```python
from build123d import *

# Parameters (mm, degrees)
BOSS_EXTRUDE2_DEPTH   = 58.42
BOSS_EXTRUDE2_2_DEPTH = 58.42
BOSS_EXTRUDE3_DEPTH   = 7.62
SKETCH6_W             = 73.66
SKETCH6_H             = 76.2
SKETCH6_W_2           = 70.104
SKETCH6_H_2           = 72.644
SKETCH6_W_3           = 63.5
SKETCH6_H_3           = 66.04
SKETCH6_W_4           = 58.42
SKETCH6_H_4           = 60.96
BOSS_EXTRUDE4_DEPTH   = 25.4
SKETCH7_W             = 73.66
SKETCH7_H             = 76.2
SKETCH7_W_2           = 70.104
SKETCH7_H_2           = 72.644
SKETCH7_W_3           = 63.5
SKETCH7_H_3           = 66.04
SKETCH7_W_4           = 58.42
SKETCH7_H_4           = 60.96
BOSS_EXTRUDE5_DEPTH   = 25.4
CHAMFER1_SIZE         = 2.773453185
CHAMFER1_SIZE_2       = 7.62
CUT_EXTRUDE3_REACH    = 158.41
SKETCH10_W            = 25.4
SKETCH10_H            = 177.72143494
SKETCH11_R            = 4.064
SKETCH11_R_2          = 2.5
BOSS_EXTRUDE6_DEPTH   = 10
SKETCH12_R            = 17
CUT_EXTRUDE4_DEPTH    = 6.5


with BuildPart() as part:
    # Sketch3 → Boss-Extrude2 (new body)
    with BuildSketch(Plane(origin=(0, 0, 0), x_dir=(0, 0, -1), z_dir=(1, 0, 0))):
        with BuildLine():
            Line((-62.063264719, -88.6355278), (-66.433917164, -94.877466378))
            ThreePointArc((-66.433917164, -94.877466378), (10.094726748, -115.383254712), (81.899935824, -81.899935824))
            Line((81.899935824, -81.899935824), (76.511782152, -76.511782152))
            ThreePointArc((76.511782152, -76.511782152), (9.430599988, -107.792251112), (-62.063264719, -88.6355278))
        make_face()
    extrude(amount=BOSS_EXTRUDE2_DEPTH)



with BuildPart() as body_2:
    # Sketch3 → Boss-Extrude2 2 (new body)
    with BuildSketch(Plane(origin=(0, 0, 0), x_dir=(0, 0, -1), z_dir=(1, 0, 0))):
        with BuildLine():
            ThreePointArc((28.018399098, -28.018399098), (3.453459151, -39.473218717), (-22.727392714, -32.458080603))
            Line((-22.727392714, -32.458080603), (-27.098045159, -38.70001918))
            ThreePointArc((-27.098045159, -38.70001918), (4.11758591, -47.064222317), (33.40655277, -33.40655277))
            Line((33.40655277, -33.40655277), (28.018399098, -28.018399098))
        make_face()
    extrude(amount=BOSS_EXTRUDE2_2_DEPTH)


with BuildPart() as part_1:
    add(part.part)

    add(body_2.part)  # Boss-Extrude3 merges body 2
    # Sketch4 → Boss-Extrude3 (add)
    with BuildSketch(Plane(origin=(58.42, 0, 0), x_dir=(0, 0, -1), z_dir=(1, 0, 0))):
        with BuildLine():
            Line((-22.727392714, -32.458080603), (-66.433917164, -94.877466378))
            ThreePointArc((-66.433917164, -94.877466378), (10.094726748, -115.383254712), (81.899935824, -81.899935824))
            Line((81.899935824, -81.899935824), (28.018399098, -28.018399098))
            ThreePointArc((28.018399098, -28.018399098), (3.453459151, -39.473218717), (-22.727392714, -32.458080603))
        make_face()
    boss_extrude3 = extrude(amount=BOSS_EXTRUDE3_DEPTH)

    # Mirror1: Boss-Extrude3 across plane
    add(boss_extrude3.mirror(Plane.ZY.offset(-29.21)))

    # Sketch6 → Boss-Extrude4 (add)
    # profile 1 of 2: a face of its own
    with BuildSketch(Plane(origin=(0, 0, 0), x_dir=(1, 0, 0), z_dir=(0, 0.5735764363510462, 0.8191520442889917))):
        with Locations((29.21, -77.724)):
            Rectangle(SKETCH6_W, SKETCH6_H)
        with Locations((29.21, -77.724)):
            Rectangle(SKETCH6_W_2, SKETCH6_H_2, mode=Mode.SUBTRACT)
    # profile 2 of 2: a face of its own
    with BuildSketch(Plane(origin=(0, 0, 0), x_dir=(1, 0, 0), z_dir=(0, 0.5735764363510462, 0.8191520442889917))):
        with Locations((29.21, -77.724)):
            Rectangle(SKETCH6_W_3, SKETCH6_H_3)
        with Locations((29.21, -77.724)):
            Rectangle(SKETCH6_W_4, SKETCH6_H_4, mode=Mode.SUBTRACT)
    extrude(amount=BOSS_EXTRUDE4_DEPTH)

    # Sketch7 → Boss-Extrude5 (add)
    # profile 1 of 2: a face of its own
    with BuildSketch(Plane(origin=(0, 0, 0), x_dir=(1, 0, 0), z_dir=(0, 0.7071067811865503, -0.7071067811865447))):
        with Locations((29.21, 77.724)):
            Rectangle(SKETCH7_W, SKETCH7_H)
        with Locations((29.21, 77.724)):
            Rectangle(SKETCH7_W_2, SKETCH7_H_2, mode=Mode.SUBTRACT)
    # profile 2 of 2: a face of its own
    with BuildSketch(Plane(origin=(0, 0, 0), x_dir=(1, 0, 0), z_dir=(0, 0.7071067811865503, -0.7071067811865447))):
        with Locations((29.21, 77.724)):
            Rectangle(SKETCH7_W_3, SKETCH7_H_3)
        with Locations((29.21, 77.724)):
            Rectangle(SKETCH7_W_4, SKETCH7_H_4, mode=Mode.SUBTRACT)
    extrude(amount=BOSS_EXTRUDE5_DEPTH)

    # Chamfer1
    # the kernel refuses this chamfer: 7.62, 2.773453185 mm, written as the material it takes off along each edge
    with BuildSketch(Plane(origin=(58.42, -15.446040528, -51.367065013), x_dir=(0, 0.7736626875489875, 0.6335977003544738), z_dir=(-1, 0, 0)), Plane(origin=(0, -24.131177697, 47.904507084), x_dir=(0, 0.8719320989550161, -0.489626811778011), z_dir=(1, 0, 0))) as chamfer1_piece_1:
        Polygon((CHAMFER1_SIZE * 0.995083363221, -CHAMFER1_SIZE * 0.0990409022559), (-CHAMFER1_SIZE_2 * 0.0990409022521, -CHAMFER1_SIZE_2 * 0.995083363182), (0, 0), align=None)
    extrude(amount=58.42, mode=Mode.SUBTRACT)
    with BuildSketch(Plane(origin=(0, -58.551269909, -94.472294394), x_dir=(0, -0.6977227871251116, 0.7163678610367485), z_dir=(1, 0, 0)), Plane(origin=(58.42, -74.066686317, 82.869726644), x_dir=(0, -0.562726836605906, -0.8266429140587307), z_dir=(-1, 0, 0))) as chamfer1_piece_2:
        Polygon((CHAMFER1_SIZE_2 * 0.999913086528, CHAMFER1_SIZE_2 * 0.0131840581986), (-CHAMFER1_SIZE * 0.0131840581992, CHAMFER1_SIZE * 0.999913086567), (0, 0), align=None)
    extrude(amount=58.42, mode=Mode.SUBTRACT)

    # Sketch10 → Cut-Extrude3 (cut, up to next)
    with BuildSketch(Plane(origin=(0, -13.973562988, -1.22252835), x_dir=(-1, 0, 0), z_dir=(0, -0.9961946980917453, -0.08715574274766034)), mode=Mode.PRIVATE) as cut_extrude3_sk1:
        with Locations((-29.21, 6.675062398)):
            Rectangle(SKETCH10_W, SKETCH10_H)
    cut_extrude3_tool1 = extrude(cut_extrude3_sk1.sketch, amount=CUT_EXTRUDE3_REACH, mode=Mode.PRIVATE) & part_1.part
    add(cut_extrude3_tool1.solids().sort_by_distance((29.21, -13.391793, -7.87219))[0], mode=Mode.SUBTRACT)

    # Sketch11 → Boss-Extrude6 (add)
    with BuildSketch(Plane.ZY.offset(7.62)):
        with BuildLine():
            Line((-25.298191602, 2.271893855), (-28.018399098, -28.018399098))
            ThreePointArc((-28.018399098, -28.018399098), (-17.287205304, -35.654086845), (-4.646100514, -39.350668686))
            Line((-4.646100514, -39.350668686), (-3.089724987, -22.01997949))
            ThreePointArc((-3.089724987, -22.01997949), (1.526343902, -17.41376085), (6.873353249, -21.146699798))
            Line((6.873353249, -21.146699798), (11.420958182, -37.942365374))
            ThreePointArc((11.420958182, -37.942365374), (17.292970019, -35.651291196), (22.727392714, -32.458080603))
            Line((22.727392714, -32.458080603), (33.130623676, -25.173659861))
            Line((33.130623676, -25.173659861), (24.517199578, 6.638292315))
            ThreePointArc((24.517199578, 6.638292315), (-2.217847157, 25.302987057), (-25.298191602, 2.271893855))
        make_face()
        Circle(SKETCH11_R, mode=Mode.SUBTRACT)
        with Locations((-17.454015953, -10.75208478)):
            Circle(SKETCH11_R_2, mode=Mode.SUBTRACT)
        with Locations((17.454015953, 10.75208478)):
            Circle(SKETCH11_R_2, mode=Mode.SUBTRACT)
    extrude(amount=-BOSS_EXTRUDE6_DEPTH)

    # Sketch12 → Cut-Extrude4 (cut)
    with BuildSketch(Plane.ZY.offset(7.62)):
        Circle(SKETCH12_R)
    extrude(amount=-CUT_EXTRUDE4_DEPTH, mode=Mode.SUBTRACT)


solid = part_1.part
```
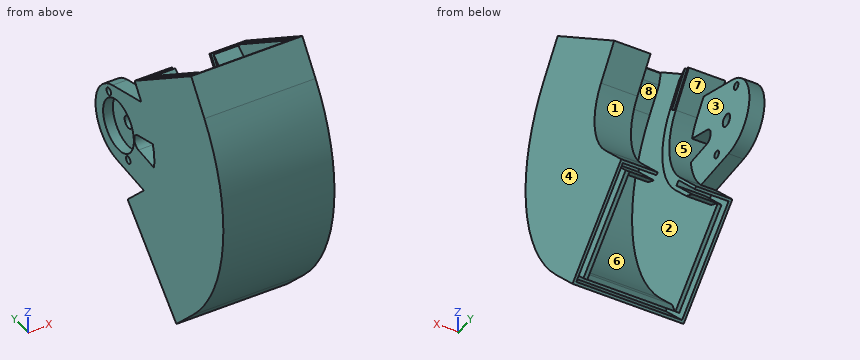
The model under review builds one solid part; all positions refer to its coordinate system, in mm. Face numbers are marked on the shaded views. A direction names the side the tool comes from. Give positions to 0.01 mm unless a question says otherwise; leave off trailing zeros. Write each loop counter-clockwise with the first axis right and the second up, starting at its lowest first coordinate (ties: lowest second). Pieces come first, ordered by that corner, then holes. Notation, with made-up numbers: M 65,-38 L 109,-38 A32 cw 109,-1 Z; hole C -10,72 d6. An arc over 180 degrees is marked long. Answer in a Markdown table with one row per item.
Item 1: Draft analysis for pull direction X (two halves, no side actions). For the marked faces 1, 2 and 3, state which applies: +X half, -X half, draft (parallel to the pull), parting line (faces both ways), or undercut.
Check sheet entries:
| item | result |
|---|---|
| face 1 | draft |
| face 2 | undercut |
| face 3 | +X half |
Item 2: Add section C-C on z = 0. Give the boundary of the cut face in (x, y).
Check sheet entries:
| item | result |
|---|---|
| outline | M -7.62,-115.82 L 66.04,-115.82 L 66.04,-39.62 L 41.91,-39.62 L 41.91,-47.24 L 58.42,-47.24 L 58.42,-108.2 L 0,-108.2 L 0,-47.24 L 16.51,-47.24 L 16.51,-39.62 L -7.62,-39.62 Z; M -7.62,-17.79 L 2.38,-17.79 L 2.38,-4.06 L -1.12,-4.06 L -1.12,-17 L -7.62,-17 Z; M -7.62,17 L -1.12,17 L -1.12,4.06 L 2.38,4.06 L 2.38,25.4 L -7.62,25.4 Z |
Item 3: Add section D-D on y = -103.5. Give the boundary of the cut face in (x, z).
Check sheet entries:
| item | result |
|---|---|
| outline | M -7.62,-51.99 L 66.04,-51.99 L 66.04,51.99 L -7.62,51.99 Z; hole M 0,-31.56 L 58.42,-31.56 L 58.42,31.56 L 0,31.56 Z |
Item 4: Add section B-B on y = 0. Give the boundary of the cut face in (x, z).
Check sheet entries:
| item | result |
|---|---|
| outline | M -7.62,-25.5 L 2.38,-25.5 L 2.38,-4.06 L -1.12,-4.06 L -1.12,-17 L -7.62,-17 Z; M -7.62,17 L -1.12,17 L -1.12,4.06 L 2.38,4.06 L 2.38,26.31 L -7.62,26.31 Z |
Item 5: For line 1 along X through (y, z) = (-35, -35.5); line 2 along X through (y, z) = (-94.5, 39); line 3 along Y through (x, z) = (-6, 0), list the stretches that pass through material, from the lowest coordinate up.
Check sheet entries:
| item | result |
|---|---|
| line 1 | -7.62 to -5.84, -2.54 to 0, 58.42 to 60.96, 64.26 to 66.04 |
| line 2 | -7.62 to 0, 58.42 to 66.04 |
| line 3 | -115.82 to -39.62, -17.79 to -17, 17 to 25.4 |
Item 6: Tool access review of the marked faces 4, 5, 6, 7 and 8: name each direction out of +Z, -Z, +X, -X, +Y, -Y from which nothing blocks a thin tool from reaching the whole face with its end or side.
Check sheet entries:
| item | result |
|---|---|
| face 4 | +Z, -Z, +X, +Y, -Y |
| face 5 | +X |
| face 6 | none |
| face 7 | +X, +Y |
| face 8 | +Y |
Item 7: For P1, Ø11, axis at y = -29, z = -8.5, coming from the +X side; P2, Ø4, axis at x = 39, z = 27.5, coming from the -Y side; P3, Ø3, axis at x = 9, z = 62.5, coming from the +Y side; P4, Ø6, axis at y = -10.75, z = -17.45, coming from the -X side, all flat-tipped, find the tip position at first contact; note any pin that passes through.
Check sheet entries:
| item | result |
|---|---|
| P1 | x = 2.38 |
| P2 | y = -112.98 |
| P3 | y = -87.28 |
| P4 | x = -7.62 |
